Build history of the part. All positions in model axes, mm. Give positions to 0.01 mm unless a question says otherwise; leave off trailing zeros. Order: outer loops, then holes, each group sorted by start corner. A loop starts at its lowest first (then second) coordinate and runs counter-clockwise, first axis right, second up. Notation, with made-up numbers: M -20.75,57 L 31.25,57 A4 ccw 31.25,64 Z; hole C -18.5,46 d3. An arc over 180 degrees is marked long. Use CSV: the item, a comma, the result in double quotes. Start each with the question number.
Item 1: Pin check, flat tips, straight feed: P1, Ø1.6, axis at x = -43, y = 0, coming from the -Z side; P2, Ø1.6, axis at x = -6.5, y = 0, coming from the -Z side; P3, Ø0.8, axis at x = -50, y = 0, coming from the +Z side. Stop position of each tip, or through.
Item 2: Band-saw the part on D-D on z = 11. Write the cut outline in (x, y), plus the area to 4 significant figures.
Item 3: Band-saw the part on B-B on z = -5. Write the cut outline in (x, y), plus the area to 3 significant figures.
Item 4: Wall check: line 1 along X through (y, z) = (0.35, -8.5); line 2 along Z through (x, y) = (35.5, -0.7); line 3 along X through (y, z) = (0.45, 17.5). Give the ranges that are in metal, low to high.
Item 5: Band-saw the part on C-C on x = -33.5. Write the cut outline in (y, z), plus the area to 3 significant figures.
Item 6: Band-saw the part on A-A on z = -14.5. Write the cut outline in (x, y) (1 decimal).
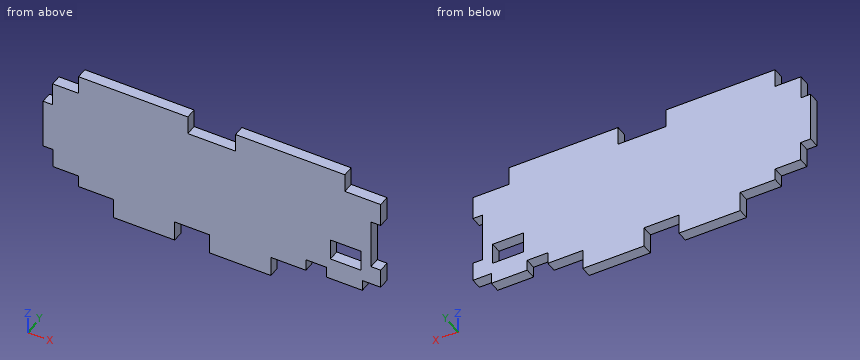
from build123d import *

# Parameters (mm, degrees)
BOSS_EXTRUDE2_DEPTH = 1.5875
SKETCH2_W           = 8.89
SKETCH2_H           = 6.223
CUT_EXTRUDE1_DEPTH  = 3.175
SKETCH4_W           = 7.3914
SKETCH4_H           = 1.27
SKETCH4_W_2         = 5.9944
SKETCH4_W_3         = 5.334
CUT_EXTRUDE2_DEPTH  = 57.051741709
SKETCH5_W           = 10.414
SKETCH5_H           = 0.635
SKETCH5_W_2         = 10.16
SKETCH5_H_2         = 0.7366
CUT_EXTRUDE3_DEPTH  = 57.051741709
SKETCH6_W           = 17.78
SKETCH6_H           = 0.254
CUT_EXTRUDE4_DEPTH  = 57.051741709
SKETCH7_W           = 10.414
SKETCH7_H           = 0.254
CUT_EXTRUDE5_DEPTH  = 56.950188363


with BuildPart() as part:
    # Sketch1 → Boss-Extrude2 (new, symmetric)
    with BuildSketch(Plane(origin=(0, 0, 0), x_dir=(1, 0, 0), z_dir=(0, 1, 0))):
        Polygon((-30.7594, 22.5171), (-30.7594, 17.0815), (-40.9194, 17.0815), (-40.9194, 14.1605), (-48.3108, 14.1605), (-48.3108, 7.3025), (-51.2318, 7.3025), (-51.2318, 0), (-51.2318, -7.3025), (-48.4124, -7.3025), (-48.4124, -14.1605), (-40.9194, -14.1605), (-40.9194, -19.5961), (-9.1694, -19.5961), (-9.1694, -14.1605), (4.699, -14.1605), (4.699, -19.5961), (36.449, -19.5961), (36.449, -14.1605), (46.863, -14.1605), (46.863, -7.3025), (44.0436, -7.3025), (44.0436, 0), (44.0436, 7.3025), (46.863, 7.3025), (46.863, 14.1605), (41.529, 14.1605), (41.529, 16.9799), (31.115, 16.9799), (31.115, 14.1605), (25.1206, 14.1605), (25.1206, 17.0815), (14.9606, 17.0815), (14.9606, 22.5171), (-2.8194, 22.5171), (-2.8194, 17.0815), (-12.9794, 17.0815), (-12.9794, 22.5171), align=None)
    extrude(amount=BOSS_EXTRUDE2_DEPTH, both=True)

    # Sketch2 → Cut-Extrude1 (cut)
    with BuildSketch(Plane(origin=(0, 1.5875, 0), x_dir=(1, 0, 0), z_dir=(0, 1, 0))):
        with Locations((36.703, 6.5786)):
            Rectangle(SKETCH2_W, SKETCH2_H)
    extrude(amount=-CUT_EXTRUDE1_DEPTH, mode=Mode.SUBTRACT)

    # Sketch4 → Cut-Extrude2 (cut, through all)
    with BuildSketch(Plane(origin=(0, 1.5875, 0), x_dir=(1, 0, 0), z_dir=(0, 1, 0))):
        with Locations((-44.6151, 13.5255)):
            Rectangle(SKETCH4_W, SKETCH4_H)
        with Locations((28.1178, 13.5255)):
            Rectangle(SKETCH4_W_2, SKETCH4_H)
        with Locations((44.196, 13.5255)):
            Rectangle(SKETCH4_W_3, SKETCH4_H)
    extrude(amount=-CUT_EXTRUDE2_DEPTH, mode=Mode.SUBTRACT)

    # Sketch5 → Cut-Extrude3 (cut, through all)
    with BuildSketch(Plane.XZ.offset(1.5875)):
        with Locations((36.322, -16.6624)):
            Rectangle(SKETCH5_W, SKETCH5_H)
        with Locations((20.0406, -16.7132)):
            Rectangle(SKETCH5_W_2, SKETCH5_H_2)
        with Locations((-7.8994, -16.7132)):
            Rectangle(SKETCH5_W_2, SKETCH5_H_2)
        with Locations((-35.8394, -16.7132)):
            Rectangle(SKETCH5_W_2, SKETCH5_H_2)
    extrude(amount=-CUT_EXTRUDE3_DEPTH, mode=Mode.SUBTRACT)

    # Sketch6 → Cut-Extrude4 (cut, through all)
    with BuildSketch(Plane.XZ.offset(1.5875)):
        with Locations((6.0706, -22.3901)):
            Rectangle(SKETCH6_W, SKETCH6_H)
        with Locations((-21.8694, -22.3901)):
            Rectangle(SKETCH6_W, SKETCH6_H)
    extrude(amount=-CUT_EXTRUDE4_DEPTH, mode=Mode.SUBTRACT)

    # Sketch7 → Cut-Extrude5 (cut, through all)
    with BuildSketch(Plane.XZ.offset(1.5875)):
        with Locations((36.322, -16.2179)):
            Rectangle(SKETCH7_W, SKETCH7_H)
    extrude(amount=-CUT_EXTRUDE5_DEPTH, mode=Mode.SUBTRACT)


solid = part.part
Model answer:
1,P1,"stops at z = -12.89"
1,P2,"stops at z = -16.34"
1,P3,"stops at z = 7.3"
2,outline,"M -48.41,-1.59 L 46.86,-1.59 L 46.86,1.59 L -48.41,1.59 Z"
2,area,"302.5 mm^2"
3,outline,"M -51.23,-1.59 L 32.26,-1.59 L 32.26,1.59 L -51.23,1.59 Z; M 41.15,-1.59 L 44.04,-1.59 L 44.04,1.59 L 41.15,1.59 Z"
3,area,"274 mm^2"
4,line 1,"x = -48.31 to 32.26, 41.15 to 46.86"
4,line 2,"z = -16.09 to -9.69, -3.47 to 19.6"
4,line 3,"x = -40.92 to -9.17, 4.7 to 36.45"
5,outline,"M -1.59,-16.34 L 1.59,-16.34 L 1.59,19.6 L -1.59,19.6 Z"
5,area,"114 mm^2"
6,outline,"M -40.9,-1.6 L 25.1,-1.6 L 25.1,1.6 L -40.9,1.6 Z; M 31.1,-1.6 L 41.5,-1.6 L 41.5,1.6 L 31.1,1.6 Z"
